Autodesk Inventor part; units mm, degrees
ref_plane "YZ Plane" through (0, 0, 0) normal (1, 0, 0) x (0, 1, 0)
ref_plane "XZ Plane" through (0, 0, 0) normal (0, 1, 0) x (-1, 0, 0)
ref_plane "XY Plane" through (0, 0, 0) normal (0, 0, 1) x (1, 0, 0)
sketch "Sketch1" plane through (0, 0, 0) normal (0, 0, 1) x (1, 0, 0)
  line L0 (0, 0) -> (8, 0)
  line L1 (8, 0) -> (8, 10)
  line L2 (8, 10) -> (0, 10)
  line L3 (0, 10) -> (0, 0)
  dimension "d0" = 8
  dimension "d1" = 10
extrude "Extrusion1" add sketch "Sketch1" along normal blind 3
sketch "Sketch2" plane through (8, 0, 0) normal (1, 0, 0) x (0, 0, -1)
  point P0 (0, 0)
sketch "Sketch3" plane through (0, 10, 0) normal (0, 1, 0) x (1, 0, 0)
  line L0 (0, 0) -> (2.95, 0)
  line L1 (2.95, 0) -> (2.95, 5)
  line L2 (2.95, 5) -> (0, 5)
  line L3 (0, 5) -> (0, 0)
  line L4 (8, 0) -> (0, 0)
  line L5 (8, 0) -> (8, -3)
  line L6 (8, 0) -> (5.05, 0)
  line L7 (5.05, 0) -> (5.05, 3)
  line L8 (5.05, 3) -> (8, 3)
  line L9 (8, 3) -> (8, 0)
  point P0 (5.05, 5)
  dimension "d4" = 2.95
  dimension "d10" = 2.95
  dimension "d11" = 3
extrude "Extrusion2" add sketch "Sketch3" against normal blind 10 contours L3 L2 L1 L0
sketch "Sketch4" plane through (8, 0, 3) normal (1, 0, 0) x (0, 0, -1)
  point P0 (3, 0)
extrude "Extrusion3" add sketch "Sketch3" against normal blind 10 contours L7 L8 L9 L4
sketch "Sketch5" plane through (8, 0, 3) normal (1, 0, 0) x (0, 0, -1)
  line L0 (3, 0) -> (3, 10)
  arc A0 (4.8073, 6.7273) -> (4.8073, 3.2727) centre (3, 5) ccw
  line L1 (4.8073, 6.7273) -> (4.8073, 3.2727)
  dimension "d14" = 5
extrude "Extrusion4" add sketch "Sketch5" along normal blind 35
sketch "Sketch6" plane through (8, 3.2727, -1.8073) normal (0, 0, -1) x (-1, 0, 0)
  line L0 (0, 3.4546) -> (0, 0)
  line L1 (0, 1.7273) -> (-30.05, 1.7273)
  circle A0 centre (-30.05, 1.7273) radius 1.45
  point P0 (8, -3.2727)
  dimension "d17" = 30.05
  dimension "d18" = 2.9
extrude "Extrusion5" add sketch "Sketch6" along normal blind 16
properties part number "Grip Stopper"
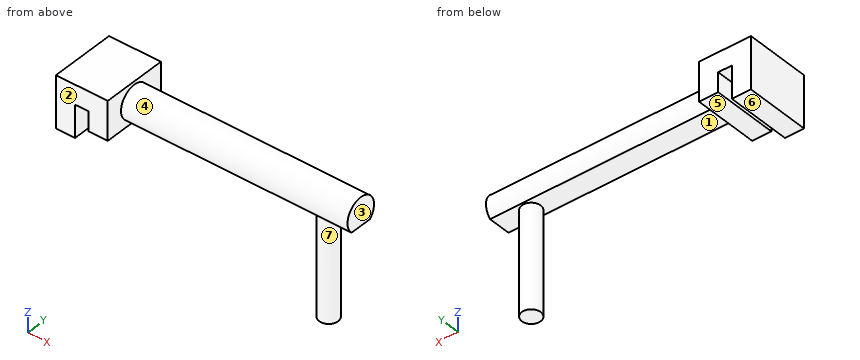
CAD build for the part. Positions are in the model's coordinates, mm. Face numbers are marked on the shaded views. A direction names the side the tool comes from. Round coordinates to 2 decimals unless told otherwise and drop trailing zeros. Loops run counter-clockwise (first coordinate to the right, second up) from the corner with the lowest first, then second, coordinate; pieces in that order, holes last.
(1) Drop flat-ended pins along their axis: pin 1 (12 mm diameter, centred on x = 35.5, z = -13.5, fed in from -Y); pin 2 (6 mm diameter, centred on y = 6.5, z = -10.5, fed in from -X); pin 3 (1.5 mm diameter, centred on x = 6, y = 4, fed in from -Z). Give the stop position or say it passes through.
(2) Cut at C-C (z = 0.5). Give the cut face in (x, y), plus the area to 3 significant figures.
(3) Which spindle directions (+Z, -Z, +X, -X, +Y, -Y) get a long thin tool onto all of the face, cutting with end or side? Do the marked faces 4, 5, 6 and 7. Say none if no direction does.
(4) Cut at B-B (x = 38.05). Give the cut face in (y, z), plus the area to 3 significant figures.
(5) Two-plate mould, pull along X, no slides. Class the marked faces 1, 2 and 3: +X half, -X half, draft (parallel to the pull), parting line (faces both ways), or undercut.
(6) Cut at A-A (y = 5). Give the cut face in (x, z), plus the area to 3 significant figures.
(7) Cut at D-D (y = 0.5). Give the cut face in (x, z), plus the area to 3 significant figures.
(8) Wall check: line 1 along Z through (x, y) = (4, 6); line 2 along X through (y, z) = (1.5, -4.5); line 3 along Y through (x, z) = (17.5, -1.5). Give the ranges that are in metal, low to high.
Findings below:
1. pin 1: stops at y = 3.55
1. pin 2: stops at x = 36.6
1. pin 3: stops at z = -3
2. outline: (0, 0) - (8, 0) - (8, 2.55) - (43, 2.55) - (43, 7.45) - (8, 7.45) - (8, 10) - (0, 10) - close
2. area: 251 mm2
3. face 4: +X
3. face 5: -Z, +Y, -Y
3. face 6: -Z, -X, +Y, -Y
3. face 7: -Z
4. outline: (3.27, -1.81) - (3.55, -1.81) - (3.55, -17.81) - (6.45, -17.81) - (6.45, -1.81) - (6.73, -1.81) arc R2.5 ccw (long way) to start
4. area: 64.4 mm2
5. face 1: undercut
5. face 2: draft
5. face 3: +X half
6. outline: (0, -5) - (2.95, -5) - (2.95, 0) - (5.05, 0) - (5.05, -3) - (8, -3) - (8, -1.81) - (36.6, -1.81) - (36.6, -17.81) - (39.5, -17.81) - (39.5, -1.81) - (43, -1.81) - (43, 2.5) - (8, 2.5) - (8, 3) - (0, 3) - close
6. area: 245 mm2
7. outline: (0, -5) - (2.95, -5) - (2.95, 0) - (5.05, 0) - (5.05, -3) - (8, -3) - (8, 3) - (0, 3) - close
7. area: 47.6 mm2
8. line 1: z = 0 to 3
8. line 2: x = 0 to 2.95
8. line 3: y = 3 to 7
